Solid Edge part; units mm, degrees
sketch "Sketch1" plane through (0, 0, 0) normal (0, 0, 1) x (1, 0, 0)
  circle A0 centre (0, 0) radius 2.413
extrude "Protrusion1" add sketch "Sketch1" along normal blind 6.35
chamfer "Chamfer1" distance 0.3619 angle 45 2 edges at (-2.413, 0, 0) (-2.413, 0, 6.35)
sketch "Sketch2" plane through (0, 0, 6.35) normal (0, 0, 1) x (1, 0, 0)
  line L0 (-0.6878, 1.1913) -> (0.6878, 1.1913)
  line L1 (1.3755, 0) -> (0.6878, 1.1913)
  line L2 (0.6878, -1.1913) -> (1.3755, 0)
  line L3 (-0.6878, -1.1913) -> (0.6878, -1.1913)
  line L4 (-1.3755, 0) -> (-0.6878, -1.1913)
  line L5 (-0.6878, 1.1913) -> (-1.3755, 0)
extrude "Cutout1" cut sketch "Sketch2" against normal blind 3.175
properties part number "24101679"
Work out the finished part from the listing and answer in its coordinate system (mm). A direction names the side the tool comes from. Give positions to 0.01 mm unless a question says otherwise; leave off trailing zeros. Loops run counter-clockwise (first coordinate to the right, second up) from the corner with the lowest first, then second, coordinate; pieces in that order, holes last. Notation, with made-up numbers: M 73,-5.5 L 128,-5.5 A26 cw 128,30.5 Z; hole C 40.25,40.5 d5. An arc over 180 degrees is marked long. One line per item, written item: value. Start each with the question number.
1. Find section C-C (z = 1.75). Give the vertices of the cut face in (x, y), and give its area (3 significant figures).
2. Each of these flat-tipped pins is pushed along its axis until it touches: P1, Ø0.7, axis at x = 0.5, z = 5, coming from the -Y side; P2, Ø1.5, axis at x = 1.5, z = 5, coming from the -Y side; P3, Ø1, axis at y = 1.5, z = 2.5, coming from the +X side. Where does it stop, or does it pass through?
3. Find section A-A (z = 3.75). Give the vertices of the cut face in (x, y).
4. Find the intervals of material crossed by probe 1 along Y at (x, z) = (0, 4.25); probe 2 along Z at (x, y) = (-0.2, -0.9) (3 decimals); probe 3 along X at (y, z) = (-0.7, 4), in increasing order.
5. Find section B-B (x = 0). Give the vertices of the cut face in (y, z) (3 decimals).
6. Which of the six approach directions +Z, -Z, +X, -X, +Y, -Y give full straight-line access (tool end or side, diameter ignored) to faces 5 (the face through (0, 0, 0)), 6 (the face through (1.03, -0.6, 4.78))?
7. Determine the mould class of faces 1 (the face through (1, -1, 6.35)), 2 (the face through (0, 0, 3.175)), 3 (the face through (-1.915, 1.468, 3.136)), 4 (the face through (-1.03, 0.6, 4.78)) for opening direction X: released by +X, released by -X, zero draft, split by the parting line, or undercut.
Reported:
1. outline: C 0,0 d4.83
1. area: 18.3 mm²
2. P1: stops at y = -2.41
2. P2: stops at y = -2.29
2. P3: stops at x = 2.2
3. outline: C 0,0 d4.83; hole M -1.38,0 L -0.69,-1.19 L 0.69,-1.19 L 1.38,0 L 0.69,1.19 L -0.69,1.19 Z
4. probe 1: y = -2.41 to -1.19, 1.19 to 2.41
4. probe 2: z = 0 to 3.175
4. probe 3: x = -2.31 to -0.97, 0.97 to 2.31
5. outline: M -2.413,0.362 L -2.051,0 L 2.051,0 L 2.413,0.362 L 2.413,5.988 L 2.051,6.35 L 1.191,6.35 L 1.191,3.175 L -1.191,3.175 L -1.191,6.35 L -2.051,6.35 L -2.413,5.988 Z
6. face 5: -Z, +X, -X, +Y, -Y
6. face 6: +Z
7. face 1: zero draft
7. face 2: undercut
7. face 3: split by the parting line
7. face 4: undercut
